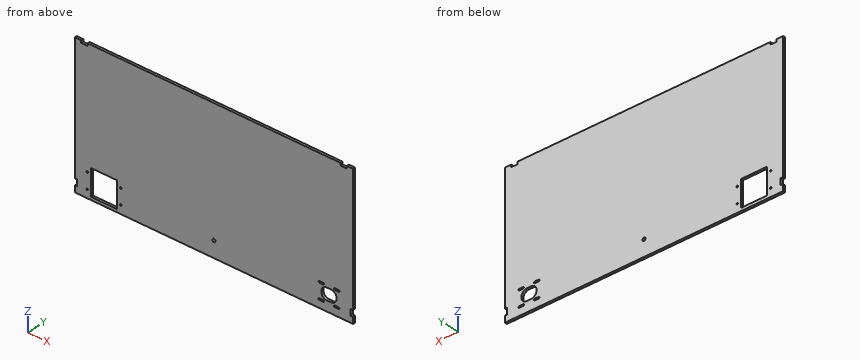
```python
from build123d import *

# Parameters (mm, degrees)
SKETCH1_R           = 3.175
BOSS_EXTRUDE1_DEPTH = 4.7625
SKETCH5_R           = 1.5875
SKETCH5_W           = 51.999999886
SKETCH5_H           = 51.999999886
CUT_EXTRUDE2_DEPTH  = 625.775544821


with BuildPart() as part:
    # Sketch1 → Boss-Extrude1 (new body)
    with BuildSketch(Plane(origin=(0, 0, 0), x_dir=(1, 0, 0), z_dir=(0, 1, 0))):
        Polygon((0, 0), (12.7, 0), (12.7, 4.7625), (25.4, 4.7625), (25.4, 0), (533.4, 0), (533.4, 4.7625), (546.1, 4.7625), (546.1, 0), (558.8, 0), (558.8, 254), (554.0375, 254), (554.0375, 266.7), (558.8, 266.7), (558.8, 279.4), (0, 279.4), (0, 266.7), (4.7625, 266.7), (4.7625, 254), (0, 254), align=None)
        with Locations(Location((279.4, 247.65, 0), (0, 0, 90))):
            Circle(SKETCH1_R, mode=Mode.SUBTRACT)
        with BuildLine():
            Line((38.9, 264.75), (46.9, 264.75))
            ThreePointArc((46.9, 264.75), (48.5, 263.15), (46.9, 261.55))
            Line((46.9, 261.55), (38.9, 261.55))
            ThreePointArc((38.9, 261.55), (37.3, 263.15), (38.9, 264.75))
        make_face(mode=Mode.SUBTRACT)
        with BuildLine():
            Line((69.9, 264.75), (77.9, 264.75))
            ThreePointArc((77.9, 264.75), (79.5, 263.15), (77.9, 261.55))
            Line((77.9, 261.55), (69.9, 261.55))
            ThreePointArc((69.9, 261.55), (68.3, 263.15), (69.9, 264.75))
        make_face(mode=Mode.SUBTRACT)
        with BuildLine():
            Line((38.9, 233.75), (46.9, 233.75))
            ThreePointArc((46.9, 233.75), (48.5, 232.15), (46.9, 230.55))
            Line((46.9, 230.55), (38.9, 230.55))
            ThreePointArc((38.9, 230.55), (37.3, 232.15), (38.9, 233.75))
        make_face(mode=Mode.SUBTRACT)
        with BuildLine():
            Line((69.9, 233.75), (77.9, 233.75))
            ThreePointArc((77.9, 233.75), (79.5, 232.15), (77.9, 230.55))
            Line((77.9, 230.55), (69.9, 230.55))
            ThreePointArc((69.9, 230.55), (68.3, 232.15), (69.9, 233.75))
        make_face(mode=Mode.SUBTRACT)
        with BuildLine():
            Line((490.9, 264.75), (498.9, 264.75))
            ThreePointArc((498.9, 264.75), (500.5, 263.15), (498.9, 261.55))
            Line((498.9, 261.55), (490.9, 261.55))
            ThreePointArc((490.9, 261.55), (489.3, 263.15), (490.9, 264.75))
        make_face(mode=Mode.SUBTRACT)
        with BuildLine():
            Line((490.9, 233.75), (498.9, 233.75))
            ThreePointArc((498.9, 233.75), (500.5, 232.15), (498.9, 230.55))
            Line((498.9, 230.55), (490.9, 230.55))
            ThreePointArc((490.9, 230.55), (489.3, 232.15), (490.9, 233.75))
        make_face(mode=Mode.SUBTRACT)
        with BuildLine():
            Line((521.9, 233.75), (529.9, 233.75))
            ThreePointArc((529.9, 233.75), (531.5, 232.15), (529.9, 230.55))
            Line((529.9, 230.55), (521.9, 230.55))
            ThreePointArc((521.9, 230.55), (520.3, 232.15), (521.9, 233.75))
        make_face(mode=Mode.SUBTRACT)
        with BuildLine():
            Line((529.9, 261.55), (521.9, 261.55))
            ThreePointArc((521.9, 261.55), (520.3, 263.15), (521.9, 264.75))
            Line((521.9, 264.75), (529.9, 264.75))
            ThreePointArc((529.9, 264.75), (531.5, 263.15), (529.9, 261.55))
        make_face(mode=Mode.SUBTRACT)
        with BuildLine():
            Line((54.4, 259.15), (62.4, 259.15))
            ThreePointArc((62.4, 259.15), (73.9, 247.65), (62.4, 236.15))
            Line((62.4, 236.15), (54.4, 236.15))
            ThreePointArc((54.4, 236.15), (42.9, 247.65), (54.4, 259.15))
        make_face(mode=Mode.SUBTRACT)
        with BuildLine():
            Line((506.4, 259.15), (514.4, 259.15))
            ThreePointArc((514.4, 259.15), (525.9, 247.65), (514.4, 236.15))
            Line((514.4, 236.15), (506.4, 236.15))
            ThreePointArc((506.4, 236.15), (494.9, 247.65), (506.4, 259.15))
        make_face(mode=Mode.SUBTRACT)
    extrude(amount=BOSS_EXTRUDE1_DEPTH)

    # Sketch5 → Cut-Extrude2 (cut, through all)
    with BuildSketch(Plane(origin=(0, 4.7625, 0), x_dir=(1, 0, 0), z_dir=(0, 1, 0))):
        with Locations(Location((24.745, 263.144, 0), (0, 0, 270))):
            Circle(SKETCH5_R)
        with Locations(Location((24.745, 232.15, 0), (0, 0, 270))):
            Circle(SKETCH5_R)
        with Locations(Location((92.055, 263.144, 0), (0, 0, 270))):
            Circle(SKETCH5_R)
        with Locations(Location((92.055, 232.15, 0), (0, 0, 270))):
            Circle(SKETCH5_R)
        with Locations((58.4, 247.65)):
            Rectangle(SKETCH5_W, SKETCH5_H)
    extrude(amount=-CUT_EXTRUDE2_DEPTH, mode=Mode.SUBTRACT)


solid = part.part
```
For this review, take the finished solid that the model builds, in its own axes (mm). Give positions to 0.01 mm unless a question says otherwise; leave off trailing zeros. Write each loop counter-clockwise with the first axis right and the second up, starting at its lowest first coordinate (ties: lowest second). Pieces come first, ordered by that corner, then holes. Notation, with made-up numbers: M 61,70 L 93,70 A20 cw 93,86 Z; hole C 82,59 d3. An arc over 180 degrees is marked long. One line per item, written item: value.
1) For line 1 (X direction, y = 2.05, z = -247.65) (3 decimals); line 2 (X direction, y = 2.5, z = -232.15); line 3 (Z direction, x = 492, y = 3.6), list the stretches that pass through material, from the lowest coordinate up. Write a range as from..to.
Results are:
line 1: x = 0..32.4, 84.4..276.225, 282.575..494.9, 525.9..558.8
line 2: x = 0..23.16, 26.33..32.4, 84.4..90.47, 93.64..489.3, 500.5..520.3, 531.5..558.8
line 3: z = -279.4..-264.75, -261.55..-233.75, -230.55..0
2) Take a section at B-B, the plane y = 2.7. Count the separate pieces of the cut face and the enclosed holes in it, then the cut area to 3 significant figures.
Results are:
separate pieces: 1
enclosed holes: 11
area: 152,000 mm²
3) Take a section at A-A, the plane x = 52. Write out the cut boundary in (y, z), then the cut area to 3 significant figures.
Results are:
outline: M 0,-279.4 L 4.76,-279.4 L 4.76,-273.65 L 0,-273.65 Z; M 0,-221.65 L 4.76,-221.65 L 4.76,0 L 0,0 Z
area: 1,080 mm²
4) For P1, Ø1.9, axis at x = 24.745, z = -263.144, coming from the -Y side; P2, Ø1.4, axis at x = 493, y = 2, coming from the +Z side; P3, Ø2.5, axis at x = 17.5, y = 2, coming from the +Z side, all flat-tipped, find the tip position at first contact; note any pin that passes through.
Results are:
P1: passes through
P2: stops at z = 0
P3: stops at z = -4.76
